Source: CAD feature listing. Evaluate the final solid. Frame: model axes, mm. Round coordinates to 2 decimals unless told otherwise and drop trailing zeros. Loops run counter-clockwise (first coordinate to the right, second up) from the corner with the lowest first, then second, coordinate; pieces in that order, holes last.
(1) Material intervals for probe 1 along X at (y, z) = (-3.5, 20.25); probe 2 along Z at (x, y) = (77, -16.5); probe 3 along X at (y, z) = (-19.5, 3), sorted ascending.
(2) Section B-B, the plane z = 14. Return the cut outline in (x, y), plus the area to 3 significant figures.
(3) Section A-A, the plane x = 40. Return the cut outline in (y, z), plus the area to 3 significant figures.
(4) First-contact query: pin 1 Ø3 at (x, y) = (57.5, -17) entering from +Z; pin 2 Ø3 at (x, z) = (120, 2) entering from +Y; pin 3 Ø7 at (y, z) = (-5.07, 14) entering from +X. Flat tips, straight axial feed; report the tip coordinate or a pass-through.
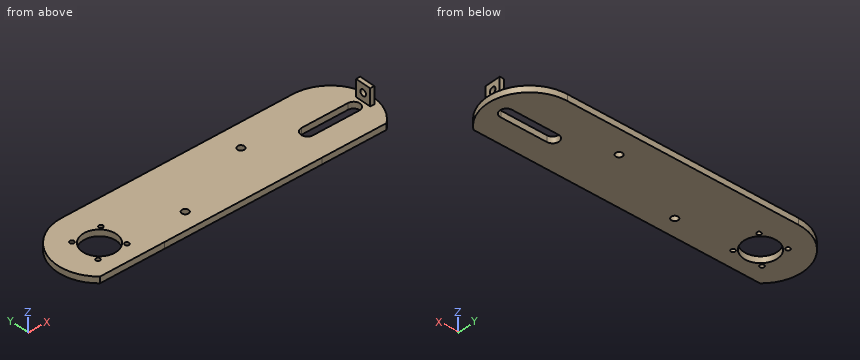
```python
from build123d import *

# Parameters (mm, degrees)
F0_R     = 3.25
F0_R_2   = 16
F1_DEPTH = 6
F2_W     = 4
F2_H     = 15
F3_DEPTH = 16
F4_R     = 3
F5_DEPTH = 25
F6_R     = 2
F6_R_2   = 16
F7_DEPTH = 25


# Not quite as in the source:
# - ends of sketch curves that miss each other by under 0.0002 mm in the source are joined


with BuildPart() as f1:
    # F0 (on Top) → F1 (new body)
    with BuildSketch(Plane.XY):
        with BuildLine():
            ThreePointArc((136.4575130484, -35.0000000549), (147.4165738824, 9.1421355849), (110, 35))
            Line((110, 35), (75, 35))
            Line((75, 35), (-75, 35))
            Line((-75, 35), (-110, 35))
            ThreePointArc((-110, 35), (-147.4165737498, 9.1421359357), (-136.4575136109, -34.9999995588))
            Line((-136.4575136109, -34.9999995588), (-75, -35))
            Line((-75, -35), (75, -35))
            Line((75, -35), (136.4575130484, -35.0000000549))
        make_face()
        with Locations((-40, -18)):
            Circle(F0_R, mode=Mode.SUBTRACT)
        with Locations((-110, -5)):
            Circle(F0_R_2, mode=Mode.SUBTRACT)
        with BuildLine():
            Line((88, 1), (132, 1))
            ThreePointArc((132, 1), (137.9996084013, -5.0685494815), (131.862909985, -10.9984336562))
            Line((131.862909985, -10.9984336562), (88.000112, -11))
            ThreePointArc((88.000112, -11), (82.0000000003, -5.000056), (88, 1))
        make_face(mode=Mode.SUBTRACT)
        with Locations((40, 12)):
            Circle(F0_R, mode=Mode.SUBTRACT)
    extrude(amount=F1_DEPTH)

    # F2 (on face) → F3 (join)
    with BuildSketch(Plane.XY.offset(6)):
        with Locations((143, -5.0685494815)):
            Rectangle(F2_W, F2_H)
    extrude(amount=F3_DEPTH)

    # F4 (on face) → F5 (cut)
    with BuildSketch(Plane.YZ.offset(145)):
        with Locations((-5.0685494815, 14)):
            Circle(F4_R)
    extrude(amount=-F5_DEPTH, mode=Mode.SUBTRACT)

    # F6 (on face) → F7 (cut)
    with BuildSketch(Plane.XY.offset(6)):
        with Locations((-123.7885822331, 8.7885822331)):
            Circle(F6_R)
        with Locations((-96.2114177669, 8.7885822331)):
            Circle(F6_R)
        with Locations((-96.2114177669, -18.7885822331)):
            Circle(F6_R)
        with Locations((-123.7885822331, -18.7885822331)):
            Circle(F6_R)
        with Locations((-110, -5)):
            Circle(F6_R_2)
    extrude(amount=-F7_DEPTH, mode=Mode.SUBTRACT)


solid = f1.part
```
Output values:
1. probe 1: x = 141 to 145
1. probe 2: z = 0 to 6
1. probe 3: x = -147.28 to -125.66, -121.92 to -116.76, -103.24 to -98.08, -94.34 to -42.88, -37.12 to 147.28
2. outline: (141, -12.57) - (145, -12.57) - (145, -8.07) - (141, -8.07) - close; (141, -2.07) - (145, -2.07) - (145, 2.43) - (141, 2.43) - close
2. area: 36.0 mm2
3. outline: (-35, 0) - (8.75, 0) - (8.75, 6) - (-35, 6) - close; (15.25, 0) - (35, 0) - (35, 6) - (15.25, 6) - close
3. area: 381 mm2
4. pin 1: stops at z = 6
4. pin 2: stops at y = 34.09
4. pin 3: stops at x = 145
